Could you check a few things on this drawing? It's one solid part, dimensions in mm from its lowest x, y, z. Round coordinates to 2 decimals unless told otherwise and drop trailing zeros. Loops run counter-clockwise (first coordinate to the right, second up) from the corner with the lowest first, then second, coordinate; pieces in that order, holes last. Notation, with made-up numbers: (57, 13.5) -> (83, 13.5) arc R11 cw to (83, 20.5) -> close; hole circle Ø9 at (45, 41). An arc over 180 degrees is marked (long way). Put each result on its own line as item: value. Start each with the question number.
1. I need wall thicknesses on line 1 (Y direction, x = 46.35, z = 1.5); line 2 (Y direction, x = 41, z = 1.25); line 3 (X direction, y = 64.5, z = 1.5). Which ranges of each line are inside material? Lowest first, please. Write a range as [from, to].
2. Imagine slicing it at D-D, the plane y = 9.5. Please give me the cut outline in (x, z), and give its area (3 significant figures).
3. Imagine slicing it at A-A, the plane x = 53. Please give me the cut outline in (y, z), and give its area (3 significant figures).
4. I'm going to push a flat-ended pin straight in: P1, Ø3, axis at x = 49, z = 4.5, coming from the -Y side. Where does the tip first touch, or does it pass through?
5. Imagine slicing it at B-B, the plane y = 50. Please give me the cut outline in (x, z), and give its area (3 significant figures).
6. Imagine slicing it at C-C, the plane z = 2.5. Please give me the cut outline in (x, y) (3 decimals).
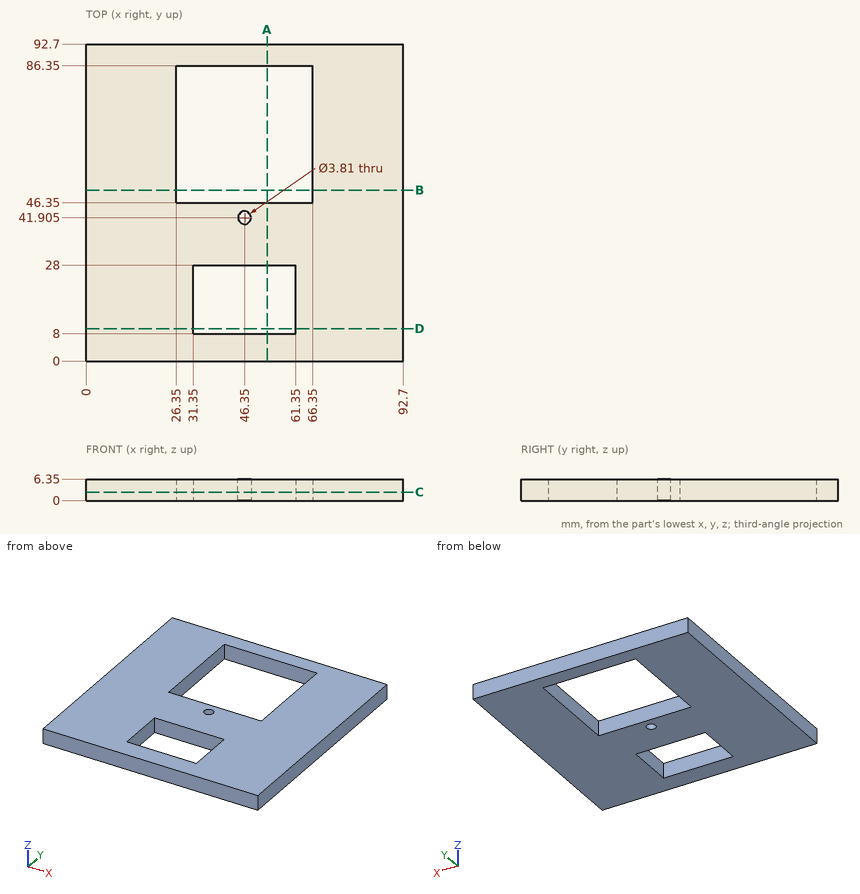
Entries:
1. line 1: [0, 8], [28, 40], [43.81, 46.35], [86.35, 92.7]
1. line 2: [0, 8], [28, 46.35], [86.35, 92.7]
1. line 3: [0, 26.35], [66.35, 92.7]
2. outline: (0, 0) -> (31.35, 0) -> (31.35, 6.35) -> (0, 6.35) -> close; (61.35, 0) -> (92.7, 0) -> (92.7, 6.35) -> (61.35, 6.35) -> close
2. area: 398 mm^2
3. outline: (0, 0) -> (8, 0) -> (8, 6.35) -> (0, 6.35) -> close; (28, 0) -> (46.35, 0) -> (46.35, 6.35) -> (28, 6.35) -> close; (86.35, 0) -> (92.7, 0) -> (92.7, 6.35) -> (86.35, 6.35) -> close
3. area: 208 mm^2
4. P1: y = 0
5. outline: (0, 0) -> (26.35, 0) -> (26.35, 6.35) -> (0, 6.35) -> close; (66.35, 0) -> (92.7, 0) -> (92.7, 6.35) -> (66.35, 6.35) -> close
5. area: 335 mm^2
6. outline: (0, 0) -> (92.7, 0) -> (92.7, 92.7) -> (0, 92.7) -> close; hole (26.35, 46.35) -> (66.35, 46.35) -> (66.35, 86.35) -> (26.35, 86.35) -> close; hole (31.35, 8) -> (61.35, 8) -> (61.35, 28) -> (31.35, 28) -> close; hole circle Ø3.81 at (46.35, 41.905)
